from build123d import *

# Parameters (mm, degrees)
SKETCH1_W           = 67
SKETCH1_H           = 145
BOSS_EXTRUDE1_DEPTH = 4
CUT_EXTRUDE1_DEPTH  = 160.781100259
SKETCH4_R           = 2.4
CUT_EXTRUDE2_DEPTH  = 160.781100259
SKETCH5_R           = 2.9
CUT_EXTRUDE3_DEPTH  = 160.781100259
FILLET1_R           = 10
FILLET2_R           = 2


with BuildPart() as part:
    # Sketch1 → Boss-Extrude1 (new body)
    with BuildSketch(Plane(origin=(0, 0, 0), x_dir=(1, 0, 0), z_dir=(0, 1, 0))):
        with Locations((33.5, 72.5)):
            Rectangle(SKETCH1_W, SKETCH1_H)
    extrude(amount=BOSS_EXTRUDE1_DEPTH)

    # Sketch2 → Cut-Extrude1 (cut, through all)
    with BuildSketch(Plane(origin=(0, 4, 0), x_dir=(1, 0, 0), z_dir=(0, 1, 0))):
        with BuildLine():
            Line((67, 78.5), (67, 93.5))
            Line((67, 93.5), (60.717797887, 93.5))
            ThreePointArc((60.717797887, 93.5), (40.5, 86), (60.717797887, 78.5))
            Line((60.717797887, 78.5), (67, 78.5))
        make_face()
    extrude(amount=-CUT_EXTRUDE1_DEPTH, mode=Mode.SUBTRACT)

    # Sketch4 → Cut-Extrude2 (cut, through all)
    with BuildSketch(Plane(origin=(0, 4, 0), x_dir=(1, 0, 0), z_dir=(0, 1, 0))):
        with Locations(Location((63.31370855, 74.68629145, 0), (0, 0, 270))):
            Circle(SKETCH4_R)
        with Locations(Location((52, 69.999999928, 0), (0, 0, 270))):
            Circle(SKETCH4_R)
        with Locations(Location((40.68629145, 74.68629145, 0), (0, 0, 270))):
            Circle(SKETCH4_R)
        with Locations(Location((40.68629145, 97.31370855, 0), (0, 0, 270))):
            Circle(SKETCH4_R)
        with Locations(Location((52, 102.000000072, 0), (0, 0, 270))):
            Circle(SKETCH4_R)
        with Locations(Location((63.31370855, 97.31370855, 0), (0, 0, 270))):
            Circle(SKETCH4_R)
    extrude(amount=-CUT_EXTRUDE2_DEPTH, mode=Mode.SUBTRACT)

    # Sketch5 → Cut-Extrude3 (cut, through all)
    with BuildSketch(Plane(origin=(0, 4, 0), x_dir=(1, 0, 0), z_dir=(0, 1, 0))):
        with Locations(Location((15, 130, 0), (0, 0, 270))):
            Circle(SKETCH5_R)
        with Locations(Location((15, 90, 0), (0, 0, 270))):
            Circle(SKETCH5_R)
        with Locations(Location((52, 10, 0), (0, 0, 270))):
            Circle(SKETCH5_R)
        with Locations(Location((15, 30, 0), (0, 0, 270))):
            Circle(SKETCH5_R)
        with Locations(Location((45, 130, 0), (0, 0, 270))):
            Circle(SKETCH5_R)
        with Locations(Location((45, 45, 0), (0, 0, 270))):
            Circle(SKETCH5_R)
    extrude(amount=-CUT_EXTRUDE3_DEPTH, mode=Mode.SUBTRACT)

    # Fillet1
    fillet1_edges = [part.edges().sort_by_distance(p)[0] for p in [
        (67, 2, -145),
    ]]
    fillet(fillet1_edges, radius=FILLET1_R)

    # Fillet2
    fillet2_edges = [part.edges().sort_by_distance(p)[0] for p in [
        (67, 2, -93.5),
        (67, 2, -78.5),
        (0, 2, -145),
        (67, 2, 0),
        (0, 2, 0),
    ]]
    fillet(fillet2_edges, radius=FILLET2_R)


solid = part.part
For this review, take the finished solid that the model builds, in its own axes (mm). Coordinates: 2 decimals unless noted, no trailing zeros. Write each loop counter-clockwise with the first axis right and the second up, starting at its lowest first coordinate (ties: lowest second). Pieces come first, ordered by that corner, then holes. Notation, with made-up numbers: (62, 60) -> (91, 60) arc R28 cw to (91, 85) -> close; hole circle Ø10 at (2, -8.75). An arc over 180 degrees is marked (long way). Write each question's results on one line, items separated by ' | '. Start each with the question number.
1) Insertion check: pin 1 (7.5 mm diameter, centred on x = 63.31, z = -97.31, fed in from -Y); pin 2 (2 mm diameter, centred on y = 2.5, z = -93.5, fed in from +X); pin 3 (1 mm diameter, centred on y = 1.5, z = -91, fed in from +X); pin 4 (1.2 mm diameter, centred on x = 63, y = 2, fed in from -Z). Each pin has a flat end and moves straight along its axis. Give the tip position at first contact, or say it passes through.
2) Consider section B-B (z = -70). Write out the cut boundary in (x, y).
3) Consider section C-C (z = -130). Write out the cut boundary in (x, y), plus the area to 3 significant figures.
4) Consider section D-D (x = 52). Write out the cut boundary in (y, z), plus the area to 3 significant figures.
5) Wall thickness on L1, parallel to Z at x = 63, y = 1.4; L2, parallel to X at y = 1.75, z = -130; L3, parallel to X at y = 2.6, z = -70: over which ranges is each line inside the solid? List them lowest first. Write a range as [from, to].
6) The part is to be moulded in two halves that separate along X. For faces 1 (the face through (63, 2, -78.5)), 2 (the face through (63.99, 2.03, -142.15)), 3 (the face through (42.71, 2.03, -96.02)), 4 (the face through (43.066, 2.028, -74.999)), say which applies: +X half, -X half, draft (parallel to the pull), parting line (faces both ways), or undercut.
7) Consider section A-A (x = 15). Write out the cut boundary in (y, z), plus the area to 3 significant figures.
Geometry says:
1) pin 1: y = 0 | pin 2: x = 66.73 | pin 3: x = 41.9 | pin 4: z = -143.42
2) outline: (0, 0) -> (49.6, 0) -> (49.6, 4) -> (0, 4) -> close; (54.4, 0) -> (67, 0) -> (67, 4) -> (54.4, 4) -> close
3) outline: (0, 0) -> (12.1, 0) -> (12.1, 4) -> (0, 4) -> close; (17.9, 0) -> (42.1, 0) -> (42.1, 4) -> (17.9, 4) -> close; (47.9, 0) -> (67, 0) -> (67, 4) -> (47.9, 4) -> close | area: 222 mm^2
4) outline: (0, -145) -> (4, -145) -> (4, -104.4) -> (0, -104.4) -> close; (0, -99.6) -> (4, -99.6) -> (4, -97.5) -> (0, -97.5) -> close; (0, -74.5) -> (4, -74.5) -> (4, -72.4) -> (0, -72.4) -> close; (0, -67.6) -> (4, -67.6) -> (4, -12.9) -> (0, -12.9) -> close; (0, -7.1) -> (4, -7.1) -> (4, 0) -> (0, 0) -> close | area: 426 mm^2
5) L1: [-143, -99.69], [-94.93, -93.5], [-78.5, -77.07], [-72.31, 0] | L2: [0, 12.1], [17.9, 42.1], [47.9, 67] | L3: [0, 49.6], [54.4, 67]
6) face 1: draft | face 2: +X half | face 3: undercut | face 4: undercut
7) outline: (0, -145) -> (4, -145) -> (4, -132.9) -> (0, -132.9) -> close; (0, -127.1) -> (4, -127.1) -> (4, -92.9) -> (0, -92.9) -> close; (0, -87.1) -> (4, -87.1) -> (4, -32.9) -> (0, -32.9) -> close; (0, -27.1) -> (4, -27.1) -> (4, 0) -> (0, 0) -> close | area: 510 mm^2
